Design review of the part built by this model. Coordinates are the model's own, in mm. A direction names the side the tool comes from. Give positions to 0.01 mm unless a question says otherwise; leave off trailing zeros. Order: outer loops, then holes, each group sorted by start corner. A loop starts at its lowest first (then second) coordinate and runs counter-clockwise, first axis right, second up.
```python
from build123d import *

# Parameters (mm, degrees)
F2_R = 0.99999


# Not quite as in the source:
# - a fillet or chamfer is up to 0.001 mm smaller than in the source, because OpenCascade refuses the exact size


with BuildPart() as f1:
    # F0 (on Front) → F1 (revolve)
    with BuildSketch(Plane.XZ):
        Polygon((4, 75), (0, 75), (0, 0), (4, 0), (4, 7), (5, 7), (5, 41), (6, 41), (6, 43), (5, 43), (5, 68), (4, 68), align=None)
    revolve(axis=Axis((0, 0, 37.5), (0, 0, -1)))

    # F2 (radius 1 in the source; OpenCascade refuses exactly that, so slightly less here)
    f2_edges = [f1.edges().sort_by_distance(p)[0] for p in [
        (-6, 0, 41),
        (-6, 0, 43),
        (6, 0, 42),
    ]]
    fillet(f2_edges, radius=F2_R)


solid = f1.part
```
1. For pin 1 (1 mm diameter, centred on y = -2.5, z = 53, fed in from -X); pin 2 (1 mm diameter, centred on y = 0, z = 59, fed in from +X); pin 3 (1.5 mm diameter, centred on x = -4.5, z = 44, fed in from +Y), all flat-tipped, find the tip position at first contact; note any pin that passes through.
Recorded:
pin 1: stops at x = -4.58
pin 2: stops at x = 5
pin 3: stops at y = 3.31
2. For line 1 along Y through (x, z) = (-3, 65.5); line 2 along Z through (x, y) = (1.25, -4.5); line 3 along Y through (x, z) = (-4, 51), list the stretches that pass through material, from the lowest coordinate up.
Recorded:
line 1: y = -4 to 4
line 2: z = 7 to 68
line 3: y = -3 to 3
3. Draft analysis for pull direction X (two halves, no side actions). For faces 4 (the face through (-0.867, 3.905, 3.549)), 5 (the face through (0, 0, 0)), state which applies: pulls with the +X half, pulls with the -X half, needs draft (parallel to the pull), parting line crosses it, or undercut.
Recorded:
face 4: parting line crosses it
face 5: needs draft
4. Take a section at C-C (z = 38). State the section outline as (x, y) points.
Recorded:
outline: circle Ø10 at (0, 0)
5. Machinability: for faces 1 (the face through (-1.08, 4.88, 24.24)), 2 (the face through (0, 0, 75)), 3 (the face through (-0.867, 3.905, 71.549)), which of the approach directions +Z, -Z, +X, -X, +Y, -Y give a long, thin tool a straight path to every point of the face, cutting with its end or side? Answer none if there is none.
Recorded:
face 1: -Z
face 2: +Z, +X, -X, +Y, -Y
face 3: +Z
